Source: CAD feature listing. Evaluate the final solid. Frame: model axes, mm. A direction names the side the tool comes from. Coordinates: 2 decimals unless noted, no trailing zeros. Order: outer loops, then holes, each group sorted by start corner. A loop starts at its lowest first (then second) coordinate and runs counter-clockwise, first axis right, second up. Notation, with made-up numbers: (78, 31.5) - (102, 31.5) arc R18 cw to (102, 41.5) - close; hole circle Ø7 at (15, -28). An arc over 180 degrees is marked (long way). One line per question, with ' | ' between items.
from build123d import *

# Parameters (mm, degrees)
BOSS_EXTRUDE1_DEPTH = 6.35
SKETCH3_W           = 19.05
SKETCH3_H           = 6.35
CUT_EXTRUDE1_DEPTH  = 6.35
SKETCH4_W           = 1.27
SKETCH4_H           = 6.35
CUT_EXTRUDE2_DEPTH  = 252.46
SKETCH5_W           = 19.05
SKETCH5_H           = 6.35
CUT_EXTRUDE3_DEPTH  = 6.35
SKETCH6_W           = 6.35
SKETCH6_H           = 25.4
SKETCH6_H_2         = 22.86
CUT_EXTRUDE4_DEPTH  = 6.35


with BuildPart() as part:
    # Sketch1 → Boss-Extrude1 (new body)
    with BuildSketch(Plane.XY):
        Polygon((0, 1.27), (-69.85, 1.27), (-76.2, 1.27), (-76.2, 252.73), (-69.85, 252.73), (0, 252.73), align=None)
    extrude(amount=BOSS_EXTRUDE1_DEPTH)

    # Sketch3 → Cut-Extrude1 (cut)
    with BuildSketch(Plane(origin=(0, 252.73, 0), x_dir=(1, 0, 0), z_dir=(0, 1, 0))):
        with Locations((-46.355, -3.175)):
            Rectangle(SKETCH3_W, SKETCH3_H)
        with Locations((-9.525, -3.175)):
            Rectangle(SKETCH3_W, SKETCH3_H)
    extrude(amount=-CUT_EXTRUDE1_DEPTH, mode=Mode.SUBTRACT)

    # Sketch4 → Cut-Extrude2 (cut, through all)
    with BuildSketch(Plane(origin=(0, 252.73, 0), x_dir=(1, 0, 0), z_dir=(0, 1, 0))):
        with Locations((-75.565, -3.175)):
            Rectangle(SKETCH4_W, SKETCH4_H)
    extrude(amount=-CUT_EXTRUDE2_DEPTH, mode=Mode.SUBTRACT)

    # Sketch5 → Cut-Extrude3 (cut)
    with BuildSketch(Plane.XZ.offset(-1.27)):
        with Locations((-46.355, 3.175)):
            Rectangle(SKETCH5_W, SKETCH5_H)
        with Locations((-9.525, 3.175)):
            Rectangle(SKETCH5_W, SKETCH5_H)
    extrude(amount=-CUT_EXTRUDE3_DEPTH, mode=Mode.SUBTRACT)

    # Sketch6 → Cut-Extrude4 (cut)
    with BuildSketch(Plane.XY.offset(6.35)):
        with Locations((-71.755, 45.72)):
            Rectangle(SKETCH6_W, SKETCH6_H)
        with Locations((-71.755, 109.22)):
            Rectangle(SKETCH6_W, SKETCH6_H)
        with Locations((-71.755, 160.02)):
            Rectangle(SKETCH6_W, SKETCH6_H)
        with Locations((-71.755, 209.55)):
            Rectangle(SKETCH6_W, SKETCH6_H_2)
    extrude(amount=-CUT_EXTRUDE4_DEPTH, mode=Mode.SUBTRACT)


solid = part.part
(1) Material intervals for L1, parallel to Y at x = -70.5, z = 5.25; L2, parallel to X at y = 167, z = 0.5; L3, parallel to Y at x = -54.5, z = 4.75, sorted ascending. Write a range as from..to.
Taken from the geometry:
L1: y = 1.27..33.02, 58.42..96.52, 121.92..147.32, 172.72..198.12, 220.98..252.73 | L2: x = -68.58..0 | L3: y = 7.62..246.38
(2) Cut plane C-C (x = -14). Return the cut outline in (y, z), and give its area (3 significant figures).
Taken from the geometry:
outline: (7.62, 0) - (246.38, 0) - (246.38, 6.35) - (7.62, 6.35) - close | area: 1,520 mm²
(3) Pull-direction query (X, two-part tool) for faces 1 (the flat face through (-72, 96.52, 3)), 2 (the flat face through (-68.58, 160, 3)), 3 (the flat face through (-36.83, 4, 3)); classes: pulls with the +X half, pulls with the -X half, needs draft (parallel to the pull), parting line crosses it, or undercut.
Taken from the geometry:
face 1: needs draft | face 2: pulls with the -X half | face 3: undercut
(4) Cut plane B-B (y = 116). Return the cut outline in (x, z).
Taken from the geometry:
outline: (-68.58, 0) - (0, 0) - (0, 6.35) - (-68.58, 6.35) - close
(5) Set-up query: faces 4 (the flat face through (-68.58, 46, 3)), 5 (the flat face through (-28, 1.27, 3)), 6 (the flat face through (-10, 7.62, 3)), 7 (the flat face through (-55.88, 250, 3)), 8 (the flat face through (-55.88, 4, 3)). Return all of +Z, -Z, +X, -X, +Y, -Y with unobstructed straight access to the full face (end or side cutting, diameter ignored); none if empty.
Taken from the geometry:
face 4: +Z, -Z, -X | face 5: +Z, -Z, +X, -X, -Y | face 6: +Z, -Z, +X, -Y | face 7: +Z, -Z, +Y | face 8: +Z, -Z, -Y
(6) Pin query (flat end, axial travel): P1, Ø1.9, axis at y = 250.5, z = 2.5, coming from the +X side; P2, Ø12, axis at x = -28, y = 176.5, coming from the -Z side. Return the tip coordinate at first contact, or that it passes through.
Taken from the geometry:
P1: stops at x = -19.05 | P2: stops at z = 0
